Source: CAD feature listing. Evaluate the final solid. Frame: model axes, mm. Face numbers are marked on the shaded views. A direction names the side the tool comes from. Give positions to 0.01 mm unless a question says otherwise; leave off trailing zeros. Order: outer loops, then holes, each group sorted by start corner. A loop starts at its lowest first (then second) coordinate and runs counter-clockwise, first axis right, second up.
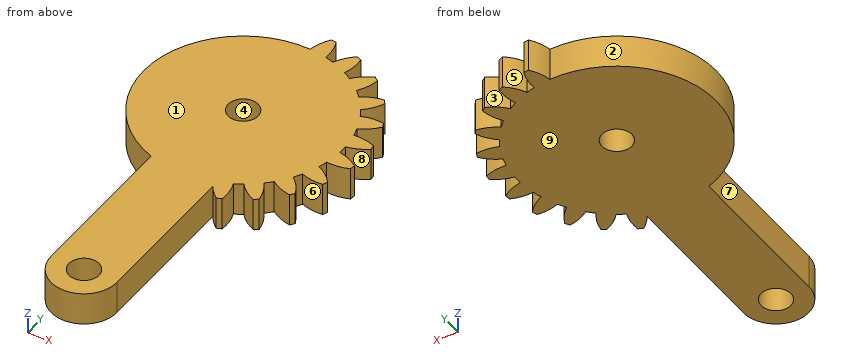
Autodesk Inventor part; units mm, degrees
ref_plane "YZ Plane" through (0, 0, 0) normal (1, 0, 0) x (0, 1, 0)
ref_plane "XZ Plane" through (0, 0, 0) normal (0, 1, 0) x (-1, 0, 0)
ref_plane "XY Plane" through (0, 0, 0) normal (0, 0, 1) x (1, 0, 0)
sketch "Náčrt1" plane through (0, 0, 0) normal (0, 0, 1) x (1, 0, 0)
  circle A0 centre (0, 0) radius 12.093
  circle A1 centre (0, 0) radius 1.825
  dimension "d0" = 24.186
  dimension "d1" = 3.65
extrude "Vysunutí1" add sketch "Náčrt1" along normal blind 4
sketch "Náčrt2" plane through (0, 0, 0) normal (0, 0, -1) x (-1, 0, 0)
  line L0 (0, 0) -> (0, 17.286)
  circle A0 centre (0, 0) radius 1.825
  line L1 (0, 0) -> (3.0566, 13.6745)
  line L2 (0, 0) -> (-0.9214, -21.9835)
  arc A1 (-0.5405, 12.0809) -> (-1.5985, 14.5344) centre (-5.8739, 11.2357) ccw
  arc A2 (-8.6515, 11.7879) -> (-9.147, 11.4077) centre (0, 0) ccw
  arc A3 (-11.4077, 9.147) -> (-11.7879, 8.6515) centre (0, 0) ccw
  arc A4 (-5.3058, 13.6254) -> (-5.8828, 13.3864) centre (0, 0) ccw
  arc A5 (-13.3864, 5.8828) -> (-13.6254, 5.3058) centre (0, 0) ccw
  arc A6 (-14.4528, 2.2177) -> (-14.5344, 1.5985) centre (0, 0) ccw
  arc A7 (-14.5344, -1.5985) -> (-14.4528, -2.2177) centre (0, 0) ccw
  arc A8 (-13.6254, -5.3058) -> (-13.3864, -5.8828) centre (0, 0) ccw
  arc A9 (-11.7879, -8.6515) -> (-11.4077, -9.147) centre (0, 0) ccw
  arc A10 (-9.147, -11.4077) -> (-8.6515, -11.7879) centre (0, 0) ccw
  arc A11 (-5.8828, -13.3864) -> (-5.3058, -13.6254) centre (0, 0) ccw
  arc A12 (-1.5985, 14.5344) -> (-2.2177, 14.4528) centre (0, 0) ccw
  circle A13 centre (0, 0) radius 12.093
  arc A14 (-2.2177, 14.4528) -> (-2.6047, 11.8091) centre (2.7657, 12.3732) ccw
  arc A15 (-5.8828, 13.3864) -> (-5.5724, 10.7326) centre (-0.5309, 12.6674) ccw
  arc A16 (-9.147, 11.4077) -> (-8.1603, 8.9247) centre (-3.7914, 12.0983) ccw
  arc A17 (-11.7879, 8.6515) -> (-10.1922, 6.5085) centre (-6.7935, 10.7048) ccw
  arc A18 (-13.6254, 5.3058) -> (-11.5294, 3.6488) centre (-9.3326, 8.5818) ccw
  arc A19 (-14.5344, 1.5985) -> (-12.0809, 0.5405) centre (-11.2357, 5.8739) ccw
  arc A20 (-14.4528, -2.2177) -> (-11.8091, -2.6047) centre (-12.3732, 2.7657) ccw
  arc A21 (-13.3864, -5.8828) -> (-10.7326, -5.5724) centre (-12.6674, -0.5309) ccw
  arc A22 (-11.4077, -9.147) -> (-8.9247, -8.1603) centre (-12.0983, -3.7914) ccw
  arc A23 (-8.6515, -11.7879) -> (-6.5085, -10.1922) centre (-10.7048, -6.7935) ccw
  arc A24 (-5.3058, -13.6254) -> (-3.6488, -11.5294) centre (-8.5818, -9.3326) ccw
  arc A25 (-3.6488, 11.5294) -> (-5.3058, 13.6254) centre (-8.5818, 9.3326) ccw
  arc A26 (-6.5085, 10.1922) -> (-8.6515, 11.7879) centre (-10.7048, 6.7935) ccw
  arc A27 (-8.9247, 8.1603) -> (-11.4077, 9.147) centre (-12.0983, 3.7914) ccw
  arc A28 (-10.7326, 5.5724) -> (-13.3864, 5.8828) centre (-12.6674, 0.5309) ccw
  arc A29 (-11.8091, 2.6047) -> (-14.4528, 2.2177) centre (-12.3732, -2.7657) ccw
  arc A30 (-12.0809, -0.5405) -> (-14.5344, -1.5985) centre (-11.2357, -5.8739) ccw
  arc A31 (-11.5294, -3.6488) -> (-13.6254, -5.3058) centre (-9.3326, -8.5818) ccw
  arc A32 (-10.1922, -6.5085) -> (-11.7879, -8.6515) centre (-6.7935, -10.7048) ccw
  arc A33 (-8.1603, -8.9247) -> (-9.147, -11.4077) centre (-3.7914, -12.0983) ccw
  arc A34 (-5.5724, -10.7326) -> (-5.8828, -13.3864) centre (-0.5309, -12.6674) ccw
  dimension "d6" = 12.6
  dimension "d17" = 169.8
  dimension "d22" = 10.8
  dimension "d29" = 150
  dimension "d33" = 150
extrude "Vysunutí2" add sketch "Náčrt2" against normal blind 4 contours A13 A14 A12 A1
pattern_circular "Kruhové pole1" count 11 over 150 about axis through (0, 0, 0) along (0, 0, -1) of "Vysunutí2"
sketch "Náčrt3" plane through (0, 0, 4) normal (0, 0, 1) x (1, 0, 0)
  line L0 (0, 0) -> (0, -30.722)
  circle A0 centre (0, -30.722) radius 1.825
  line L1 (-4, 1.3777) -> (-4, -30.722)
  line L2 (4, 1.3777) -> (4, -30.722)
  arc A1 (-4, -30.722) -> (4, -30.722) centre (0, -30.722) ccw
  line L3 (-4, -8.9953) -> (4, -8.9953)
  point P0 (-4, -33.1583)
  point P1 (4, -33.1583)
  dimension "d40" = 30.722
  dimension "d41" = 3.65
  dimension "d42" = 34.536
  dimension "d43" = 4
  dimension "d44" = 8
extrude "Vysunutí3" add sketch "Náčrt3" against normal blind 4
properties part number "zubate_kolo1" material "ABS Plastic"
1) First-contact query: pin 1 Ø3 at (x, y) = (0, 0) entering from -Z; pin 2 Ø1.2 at (y, z) = (-25, 3) entering from +X; pin 3 Ø1 at (y, z) = (-2.5, 3.5) entering from -X. Flat tips, straight axial feed; report the tip coordinate or a pass-through.
Checks:
pin 1: passes through
pin 2: stops at x = 4
pin 3: stops at x = -11.93
2) Ray query, L1, parallel to Y at x = 0, z = 1.65 (3 decimals); L2, parallel to X at y = -18, z = 2.45; L3, parallel to Y at x = -1, z = 0.35. Return the intervals inside material, ascending.
Checks:
L1: y = -34.722 to -32.547, -28.897 to -1.825, 1.825 to 12.093
L2: x = -4 to 4
L3: y = -34.59 to -32.25, -29.2 to -1.53, 1.53 to 12.05
3) Section query C-C on z = 3.1. State how many separate pieces and enclosed holes the cut face has, and give its area (3 significant figures).
Checks:
separate pieces: 1
enclosed holes: 2
area: 659 mm2
4) Section query D-D on y = -30. Output: boundary loops of the cut face in (x, z).
Checks:
outline: (-4, 0) - (-1.68, 0) - (-1.68, 4) - (-4, 4) - close; (1.68, 0) - (4, 0) - (4, 4) - (1.68, 4) - close
5) Section query B-B on y = 0. Output: boundary loops of the cut face in (x, z) (3 decimals).
Checks:
outline: (-12.093, 0) - (-1.825, 0) - (-1.825, 4) - (-12.093, 4) - close; (1.825, 0) - (12.093, 0) - (12.093, 4) - (1.825, 4) - close
6) Pull-direction query (Y, two-part tool) for the marked faces 1, 2, 3 and 4; classes: +Y half, -Y half, draft (parallel to the pull), parting line (faces both ways), or undercut.
Checks:
face 1: draft
face 2: parting line
face 3: +Y half
face 4: undercut
7) Section query A-A on x = 0. Output: boundary loops of the cut face in (y, z) (3 decimals).
Checks:
outline: (-34.722, 0) - (-32.547, 0) - (-32.547, 4) - (-34.722, 4) - close; (-28.897, 0) - (-1.825, 0) - (-1.825, 4) - (-28.897, 4) - close; (1.825, 0) - (12.093, 0) - (12.093, 4) - (1.825, 4) - close
8) Reachability of the marked faces 5, 6, 7, 8 and 9 from +Z, -Z, +X, -X, +Y, -Y: full face, straight path, thin tool, end or side. Return the list, or none.
Checks:
face 5: +Z, -Z, +Y
face 6: +Z, -Z
face 7: +Z, -Z, -X, -Y
face 8: +Z, -Z, +X
face 9: -Z, +X, -X, +Y, -Y
